Autodesk Inventor part; units mm, degrees
ref_plane "YZ Plane" through (0, 0, 0) normal (1, 0, 0) x (0, 1, 0)
ref_plane "XZ Plane" through (0, 0, 0) normal (0, 1, 0) x (-1, 0, 0)
ref_plane "XY Plane" through (0, 0, 0) normal (0, 0, 1) x (1, 0, 0)
sketch "Sketch1" plane through (0, 0, 0) normal (0, 0, 1) x (1, 0, 0)
  circle A0 centre (13.2988, -6.9384) radius 3.6
  circle A1 centre (-12.6582, -8.0479) radius 3.6
  circle A2 centre (-0.6406, 14.9863) radius 3.5
  circle A3 centre (0, 0) radius 7.5
  circle A4 centre (0, 0) radius 21.25
  point P0 (0, 0)
  dimension "d11" = 42.5
extrude "Extrusion1" add sketch "Sketch1" along normal blind 3.5
sketch "Sketch3" plane through (0, 0, 0) normal (0, 0, -1) x (-1, 0, 0)
  circle A0 centre (0, 0) radius 20.25
  dimension "d14" = 40.5
extrude "Extrusion4" cut sketch "Sketch3" against normal blind 1
properties part number "Inner disc of housing of gearbox"
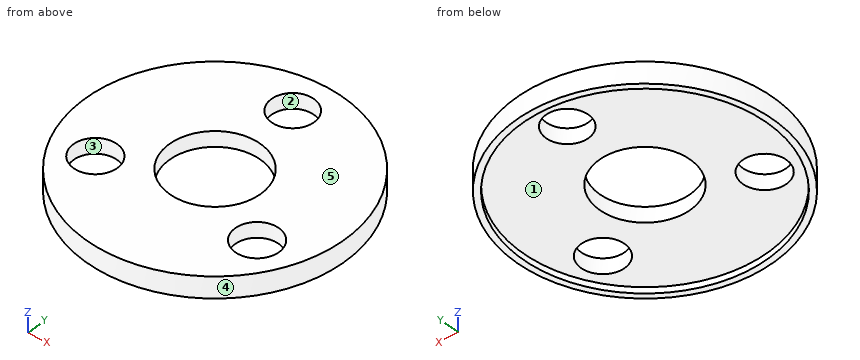
Part model, mm, in its own coordinate system. Face numbers are marked on the shaded views. A direction names the side the tool comes from. Give positions to 0.01 mm unless a question says otherwise; leave off trailing zeros. Write each loop counter-clockwise with the first axis right and the second up, starting at its lowest first coordinate (ties: lowest second). Pieces come first, ordered by that corner, then holes.
1) Two-plate mould, pull along X, no slides. Class the marked faces 3, 4 and 5: released by +X, released by -X, zero draft, split by the parting line, or undercut.
Resolved:
face 3: undercut
face 4: split by the parting line
face 5: zero draft
2) Cut at D-D on z = 1.5. Write the cut outline in (x, y), then the cut area to 3 significant figures.
Resolved:
outline: circle Ø42.5 at (0, 0); hole circle Ø7.2 at (-12.66, -8.05); hole circle Ø15 at (0, 0); hole circle Ø7 at (-0.64, 14.99); hole circle Ø7.2 at (13.3, -6.94)
area: 1,120 mm2
3) Which spindle directions (+Z, -Z, +X, -X, +Y, -Y) get a long thin tool onto all of the face, cutting with end or side? Do the marked faces 1 and 2. Say none if no direction does.
Resolved:
face 1: -Z
face 2: +Z, -Z
4) Cut at B-B on x = -3. Write the cut outline in (y, z).
Resolved:
outline: (-21.04, 0) - (-20.03, 0) - (-20.03, 1) - (-6.87, 1) - (-6.87, 3.5) - (-21.04, 3.5) - close; (6.87, 1) - (12.4, 1) - (12.4, 3.5) - (6.87, 3.5) - close; (17.57, 1) - (20.03, 1) - (20.03, 0) - (21.04, 0) - (21.04, 3.5) - (17.57, 3.5) - close
5) Cut at A-A on y = 0. Write the cut outline in (x, z).
Resolved:
outline: (-21.25, 0) - (-20.25, 0) - (-20.25, 1) - (-7.5, 1) - (-7.5, 3.5) - (-21.25, 3.5) - close; (7.5, 1) - (20.25, 1) - (20.25, 0) - (21.25, 0) - (21.25, 3.5) - (7.5, 3.5) - close
6) Cut at C-C on x = 7. Write the cut outline in (y, z), then the cut area to 3 significant figures.
Resolved:
outline: (-20.06, 0) - (-19, 0) - (-19, 1) - (-2.69, 1) - (-2.69, 3.5) - (-20.06, 3.5) - close; (2.69, 1) - (19, 1) - (19, 0) - (20.06, 0) - (20.06, 3.5) - (2.69, 3.5) - close
area: 89.0 mm2
7) Probe L1, parallel to X at y = -10, z = 2.35; L2, parallel to Z at x = 11, y = -3; L3, parallel to Y at x = 2, z = 3.15. List the from-to ranges inside material, lowest first.
Resolved:
L1: x = -18.75 to -15.68, -9.63 to 11.4, 15.19 to 18.75
L2: z = 1 to 3.5
L3: y = -21.16 to -7.23, 7.23 to 12.69, 17.28 to 21.16
8) Pin check, flat tips, straight feed: pin 1 (9.5 mm diameter, centred on x = 13.3, y = -6.94, fed in from -Z); pin 2 (1.5 mm diameter, centred on y = -8.5, z = 2.5, fed in from -X); pin 3 (1.5 mm diameter, centred on y = -7, z = 1.5, fed in from -X); pin 4 (5 mm diameter, centred on x = -1, y = -5, fed in from +Z). Stop position of each tip, or through.
Resolved:
pin 1: stops at z = 1
pin 2: stops at x = -19.79
pin 3: stops at x = -20.31
pin 4: stops at z = 3.5
